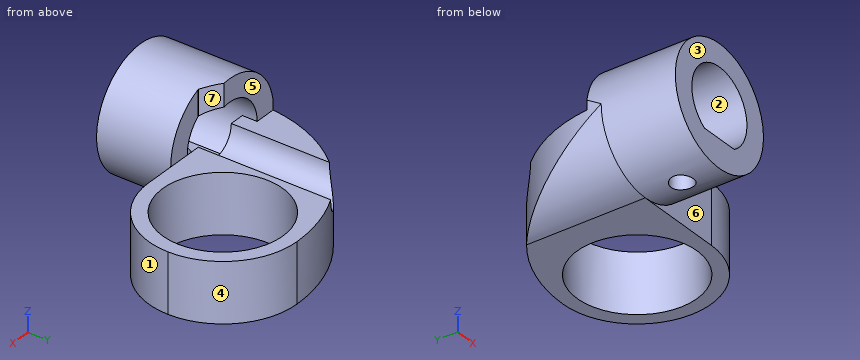
```python
from build123d import *

# Parameters (mm, degrees)
SKETCH_1_R          = 4
EXTRUDE_1_DEPTH     = 6
CUT_EXTRUDE_1_DEPTH = 9.246211251
SKETCH_4_W          = 15
SKETCH_4_H          = 10
EXTRUDE_2_DEPTH     = 4
SKETCH_5_R          = 4.05
CUT_EXTRUDE_3_DEPTH = 20.02629759
FILLET_1_R          = 10
FILLET_2_R          = 5
CUT_EXTRUDE_4_DEPTH = 16.394804409
SKETCH_7_R          = 1.5
CUT_EXTRUDE_5_DEPTH = 20.02629769
SKETCH_8_R          = 0.75
CUT_EXTRUDE_7_DEPTH = 3
SKETCH_9_W          = 2.5
SKETCH_9_H          = 1
CUT_EXTRUDE_8_DEPTH = 20.02629769
CHAMFER_1_SIZE      = 1


# Some blends are built 0.0001 mm under size
with BuildPart() as part:
    # 草图1 → 凸台-拉伸1 (new body)
    with BuildSketch(Plane(origin=(0, 0, 0), x_dir=(1, 0, 0), z_dir=(0, 1, 0))):
        with Locations(Location((0, 0, 0), (0, 0, 270))):
            Circle(SKETCH_1_R)
    extrude(amount=EXTRUDE_1_DEPTH)

    # 草图2 → 切除-拉伸1 (cut, through all)
    with BuildSketch(Plane(origin=(0, 0, 0), x_dir=(1, 0, 0), z_dir=(0, 1, 0))):
        with BuildLine():
            Line((-1.356465997, 2.1), (1.356465997, 2.1))
            ThreePointArc((1.356465997, 2.1), (0, -2.5), (-1.356465997, 2.1))
        make_face()
    extrude(amount=CUT_EXTRUDE_1_DEPTH, mode=Mode.SUBTRACT)

    # 草图4 → 凸台-拉伸2 (add)
    with BuildSketch(Plane.XY.offset(-4)):
        with Locations((3.5, 10)):
            Rectangle(SKETCH_4_W, SKETCH_4_H)
    extrude(amount=EXTRUDE_2_DEPTH)

    # 草图5 → 切除-拉伸3 (cut, through all)
    with BuildSketch(Plane.XY):
        with Locations((6, 10)):
            Circle(SKETCH_5_R)
    extrude(amount=-CUT_EXTRUDE_3_DEPTH, mode=Mode.SUBTRACT)

    # 圆角1
    # the kernel refuses this fillet: 10 mm, written as the material it takes off along each edge
    with BuildSketch(Plane(origin=(-4, 15, -29), x_dir=(0, -1, 0), z_dir=(0, 0, 1))) as fillet_1_piece_1:
        with BuildLine():
            CenterArc((FILLET_1_R, FILLET_1_R), FILLET_1_R, 180, 90)
            Line((0, FILLET_1_R), (0, 0))
            Line((0, 0), (FILLET_1_R, 0))
        make_face()
    extrude(amount=54, mode=Mode.SUBTRACT)

    # 圆角2
    fillet_2_edges = [part.edges().sort_by_distance(p)[0] for p in [
        (11, 5, -2),
        (11, 15, -2),
    ]]
    fillet(fillet_2_edges, radius=FILLET_2_R - 0.0001)  # a hair under: the kernel refuses the full size

    # 草图6 → 切除-拉伸4 (cut, through all)
    with BuildSketch(Plane.XZ.offset(-5)):
        with BuildLine():
            Line((-4, -4), (-4, 0))
            ThreePointArc((-4, 0), (-2.828427125, -2.828427125), (0, -4))
            Line((0, -4), (-4, -4))
        make_face()
    extrude(amount=-CUT_EXTRUDE_4_DEPTH, mode=Mode.SUBTRACT)

    # 草图7 → 切除-拉伸5 (cut, through all)
    with BuildSketch(Plane.XZ):
        Circle(SKETCH_7_R)
    extrude(amount=-CUT_EXTRUDE_5_DEPTH, mode=Mode.SUBTRACT)

    # 草图8 → 切除-拉伸7 (cut)
    with BuildSketch(Plane.XY.offset(-4)):
        with Locations(Location((0, 2.5, 0), (0, 0, 270))):
            Circle(SKETCH_8_R)
    extrude(amount=CUT_EXTRUDE_7_DEPTH, mode=Mode.SUBTRACT)

    # 草图9 → 切除-拉伸8 (cut, through all)
    with BuildSketch(Plane.XY):
        with Locations((2.75, 5.5)):
            Rectangle(SKETCH_9_W, SKETCH_9_H)
    extrude(amount=CUT_EXTRUDE_8_DEPTH, mode=Mode.SUBTRACT)

    # 倒角1
    chamfer_1_edges = [part.edges().sort_by_distance(p)[0] for p in [
        (1.5, 6, 2.854049622),
    ]]
    chamfer(chamfer_1_edges, length=CHAMFER_1_SIZE - 0.0001)  # a hair under: the kernel refuses the full size


solid = part.part
```
Source: CAD feature listing. Evaluate the final solid. Frame: model axes, mm. Face numbers are marked on the shaded views. A direction names the side the tool comes from. Round coordinates to 2 decimals unless told otherwise and drop trailing zeros. Loops run counter-clockwise (first coordinate to the right, second up) from the corner with the lowest first, then second, coordinate; pieces in that order, holes last.
1. Access query for the marked faces 4, 5, 6 and 7. Directions: +Z, -Z, +X, -X, +Y, -Y. A direction counts if a zero-diameter tool reaches every point of the face in a straight line with its end or side. Return the directions, or none.
2. Mould query, pull axis X, two halves, no side actions, for the marked faces 1, 2 and 3. Classes: released by +X, released by -X, zero draft, split by the parting line, or undercut.
3. Section query A-A on x = 7.5. Output: boundary loops of the cut face in (y, z).
4. Contact query for flat-ended pins moving along their axis: pin 1 (5 mm diameter, centred on x = 6.5, y = 11.5, fed in from +Z); pin 2 (2 mm diameter, centred on x = -2, y = 2, fed in from +Z); pin 3 (1.3 mm diameter, centred on x = 3, z = 1, fed in from +Y); pin 4 (5 mm diameter, centred on x = 5, y = 9, fed in from +Z). Output: stop coordinate, or through.
5. Ray query, L1, parallel to Y at x = 0, z = -2.55; L2, parallel to X at y = 10.75, z = -1; L3, parallel to Y at x = 6, z = -2.05. Return the intervals inside material, ascending.
6. Section query C-C on y = 10.5. Output: boundary loops of the cut face in (x, z).
7. Section query D-D on z = 1. Output: boundary loops of the cut face in (x, y).
8. Section query B-B on z = -0.75. Give the number of separate pieces and of enclosed holes in the cut face, and give its area (3 significant figures).
Answers below:
1. face 4: +Z, -Z, +X, +Y
1. face 5: +Z, +X, -X, +Y
1. face 6: -Z, +X, -Y
1. face 7: +Z, +X, +Y
2. face 1: released by +X
2. face 2: undercut
2. face 3: zero draft
3. outline: (5.23, -4) - (6.24, -4) - (6.24, 0) - (5.23, 0) - close; (13.76, -4) - (14.77, -4) - (14.77, 0) - (13.76, 0) - close
4. pin 1: stops at z = 0
4. pin 2: stops at z = 3.87
4. pin 3: stops at y = 5
4. pin 4: passes through
5. L1: y = 0 to 1.75, 3.25 to 13
5. L2: x = -2.18 to -1.12, 1.12 to 2.02, 9.98 to 10.94
5. L3: y = 5 to 5.95, 14.05 to 15
6. outline: (-2.35, -3.24) arc R4 ccw to (0, -4) - (1.98, -4) - (1.98, 0) - (1.5, 0) arc R1.5 cw to (-1.5, 0) - (-2.35, 0) - close; (10.02, -4) - (10.97, -4) - (10.97, 0) - (10.02, 0) - close
7. outline: (-3.87, 0) - (-2.29, 0) - (-2.29, 6) - (-3.87, 6) - close; (2.29, 0) - (3.87, 0) - (3.87, 5) - (2.29, 5) - close
8. separate pieces: 2
8. enclosed holes: 1
8. area: 61.0 mm2
